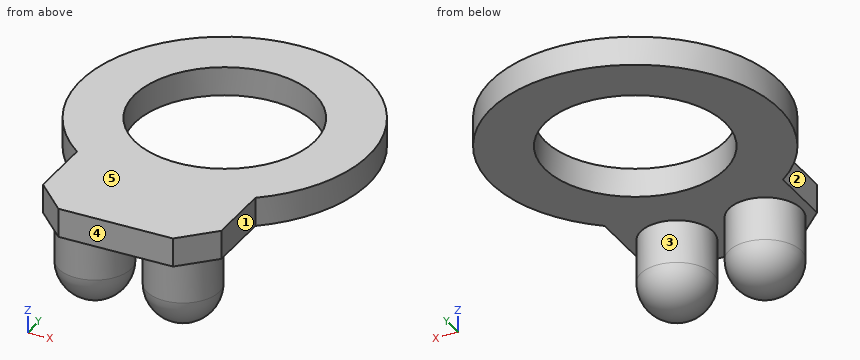
```python
from build123d import *

# Parameters (mm, degrees)
SKETCH1_R           = 5
SKETCH1_R_2         = 2
BOSS_EXTRUDE1_DEPTH = 1.6
BOSS_EXTRUDE2_START = -6
SKETCH2_R           = 2
BOSS_EXTRUDE2_DEPTH = 6
FILLET1_R           = 2


with BuildPart() as part:
    # Sketch1 → Boss-Extrude1 (new body)
    with BuildSketch(Plane.XY):
        with BuildLine():
            Line((4.95, -9.932233047), (4.95, -6.284703653))
            ThreePointArc((4.95, -6.284703653), (0, 8), (-4.95, -6.284703653))
            Line((-4.95, -6.284703653), (-4.95, -9.932233047))
            Line((-4.95, -9.932233047), (-3.182233047, -11.7))
            Line((-3.182233047, -11.7), (3.182233047, -11.7))
            Line((3.182233047, -11.7), (4.95, -9.932233047))
        make_face()
        Circle(SKETCH1_R, mode=Mode.SUBTRACT)
        with Locations((2.45, -9.2)):
            Circle(SKETCH1_R_2, mode=Mode.SUBTRACT)
        with Locations((-2.45, -9.2)):
            Circle(SKETCH1_R_2, mode=Mode.SUBTRACT)
    extrude(amount=BOSS_EXTRUDE1_DEPTH)

    # Sketch2 → Boss-Extrude2 (add)
    with BuildSketch(Plane.XY.offset(1.6).offset(BOSS_EXTRUDE2_START)):
        with Locations((2.45, -9.2)):
            Circle(SKETCH2_R)
        with Locations((-2.45, -9.2)):
            Circle(SKETCH2_R)
    extrude(amount=BOSS_EXTRUDE2_DEPTH)

    # Fillet1
    fillet1_edges = [part.edges().sort_by_distance(p)[0] for p in [
        (-4.45, -9.2, -4.4),
        (0.45, -9.2, -4.4),
    ]]
    fillet(fillet1_edges, radius=FILLET1_R)


solid = part.part
```
Design review of the part built by this model. Coordinates are the model's own, in mm. Face numbers are marked on the shaded views. A direction names the side the tool comes from. Coordinates: 2 decimals unless noted, no trailing zeros. Order: outer loops, then holes, each group sorted by start corner. A loop starts at its lowest first (then second) coordinate and runs counter-clockwise, first axis right, second up. Notation, with made-up numbers: (86.25, 89) -> (121.25, 89) arc R22 ccw to (121.25, 110) -> close; hole circle Ø5 at (55.25, -18.5). An arc over 180 degrees is marked (long way). One line per item, written item: value. Start each with the question number.
Q1. Tool access review of the marked faces 1, 2, 3, 4 and 5: name each direction out of +Z, -Z, +X, -X, +Y, -Y from which nothing blocks a thin tool from reaching the whole face with its end or side.
Q2. For probe 1 along Y at (x, z) = (0, 0.5); probe 2 along Z at (x, y) = (0.25, -9); probe 3 along X at (y, z) = (-8.25, -2.2), list the stretches that pass through material, from the lowest coordinate up.
Q3. Take a section at A-A, the plane y = 0. State the section outline as (x, z) points, then the cut area to 3 significant figures.
Q4. Take a section at B-B, the plane x = 0. State the section outline as (y, z) points, then the cut area to 3 significant figures.
Q5. Insertion check: pin 1 Ø3 at (y, z) = (-7.5, -3) entering from +X; pin 2 Ø1.3 at (y, z) = (-9, 0.5) entering from -X; pin 3 Ø1.8 at (y, z) = (-8, 1) entering from +X; pin 4 Ø4 at (x, y) = (-4, -0.5) entering from +Z. Each pin has a flat end and moves straight along its axis. Give the tip position at first contact, or say it passes through.
Q6. Take a section at D-D, the plane y = -6.75. State the section outline as (x, z) points, then the cut area to 3 significant figures.
Q7. Take a section at C-C, the plane z = -0.8. State the section outline as (x, y) points, then the cut area to 3 significant figures.
Values follow:
1. face 1: +Z, -Z, +X, -Y
1. face 2: +Z, -Z, -X, -Y
1. face 3: -Z
1. face 4: +Z, -Z, +X, -X, -Y
1. face 5: +Z, +X, -X, +Y, -Y
2. probe 1: y = -11.7 to -5, 5 to 8
2. probe 2: z = 0 to 1.6
2. probe 3: x = -4.21 to -0.69, 0.69 to 4.21
3. outline: (-8, 0) -> (-5, 0) -> (-5, 1.6) -> (-8, 1.6) -> close; (5, 0) -> (8, 0) -> (8, 1.6) -> (5, 1.6) -> close
3. area: 9.60 mm2
4. outline: (-11.7, 0) -> (-5, 0) -> (-5, 1.6) -> (-11.7, 1.6) -> close; (5, 0) -> (8, 0) -> (8, 1.6) -> (5, 1.6) -> close
4. area: 15.5 mm2
5. pin 1: stops at x = 4.43
5. pin 2: stops at x = -4.95
5. pin 3: stops at x = 4.95
5. pin 4: stops at z = 1.6
6. outline: (-4.95, 0) -> (4.95, 0) -> (4.95, 1.6) -> (-4.95, 1.6) -> close
6. area: 15.8 mm2
7. outline: circle Ø4 at (-2.45, -9.2); circle Ø4 at (2.45, -9.2)
7. area: 25.1 mm2
